For this review, take the finished solid that the model builds, in its own axes (mm). Face numbers are marked on the shaded views. A direction names the side the tool comes from. Coordinates: 2 decimals unless noted, no trailing zeros. Order: outer loops, then holes, each group sorted by start corner. A loop starts at its lowest first (then second) coordinate and runs counter-clockwise, first axis right, second up. Notation, with made-up numbers: (24, -14.5) -> (83, -14.5) arc R38 ccw to (83, 24.5) -> close; hole circle Ø2 at (87.5, -25.75). An arc over 180 degrees is marked (long way). Answer as a JSON object with one key per item and string values. Group by question number.
1) Wall thickness on L1, parallel to Y at x = -27.5, z = -1; L2, parallel to Y at x = -47.5, z = -0.75; L3, parallel to Z at x = -64, y = -17.5: over which ranges is each line inside the solid? List them lowest first.
2) Add section A-A, the plane x = -45. Write out the cut boundary in (y, z), then the cut area to 3 significant figures.
3) Add section B-B, the plane x = 8.5. Write out the cut boundary in (y, z).
4) Machinability: for the marked faces 1 and 2, which of the approach directions +Z, -Z, +X, -X, +Y, -Y give a long, thin tool a straight path to every point of the face, cutting with its end or side? Answer none if there is none.
5) Draft analysis for pull direction Y (two halves, no side actions). For the marked faces 3, 4 and 5, state which applies: +Y half, -Y half, draft (parallel to the pull), parting line (faces both ways), or undercut.
6) Add section C-C, the plane y = -19. Write out the cut boundary in (x, z).
7) For pin 1 (10.5 mm diameter, centred on x = -19.5, y = 22.5, fed in from +Z); pin 2 (1.6 mm diameter, centred on x = -50.5, z = -12.5, fed in from -Y); pin 3 (18.5 mm diameter, centred on x = 9, y = 35.5, fed in from -Z), all flat-tipped, find the tip position at first contact; note any pin that passes through.
8) Add section D-D, the plane x = -12. Write out the cut boundary in (y, z), then the cut area to 3 significant figures.
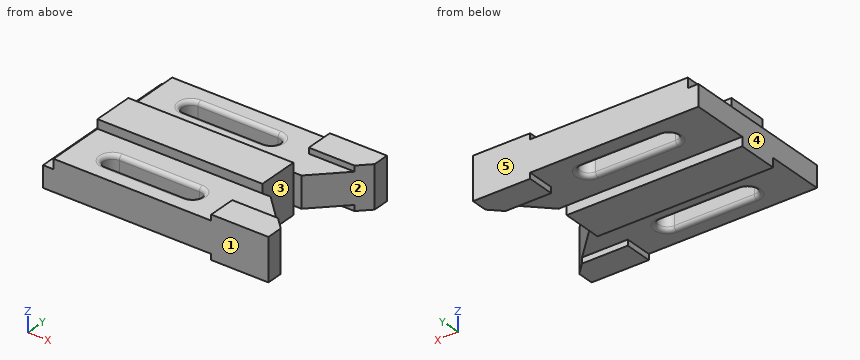
from build123d import *

# Parameters (mm, degrees)
EXTRUDE_1_DEPTH      = 9.5
EXTRUDE_2_DEPTH      = 3.5
EXTRUDE_2_DEPTH_BACK = 22.5
EXTRUDE_3_DEPTH      = 5.5
EXTRUDE_3_DEPTH_BACK = 24.5
SKETCH_8_W           = 107.5
SKETCH_8_H           = 25
SKETCH_9_W           = 6.5
SKETCH_9_H           = 96
CUT_EXTRUDE_1_DEPTH  = 11.5
CUT_EXTRUDE_2_DEPTH  = 52.5
FILLET_1_R           = 2.5


with BuildPart() as part:
    # 草图1 → 凸台-拉伸1 (new, symmetric)
    with BuildSketch(Plane.XY):
        Polygon((-107.5, 48), (30.5, 48), (30.5, 38), (5, 12.5), (0, 12.5), (0, -12.5), (5, -12.5), (30.5, -38), (30.5, -48), (-107.5, -48), align=None)
    extrude(amount=EXTRUDE_1_DEPTH, both=True)

    # 草图2 → 凸台-拉伸2 (add, two sides: drawn at the far end of the back side and taken through both)
    with BuildSketch(Plane.XY.offset(9.5).offset(-EXTRUDE_2_DEPTH_BACK)):
        Polygon((-4.5, 31), (23.5, 31), (30.5, 38), (30.5, 48), (-4.5, 48), align=None)
        Polygon((30.5, -38), (23.5, -31), (-4.5, -31), (-4.5, -48), (30.5, -48), align=None)
    extrude(amount=EXTRUDE_2_DEPTH + EXTRUDE_2_DEPTH_BACK)

    # 草图8 → 凸台-拉伸3 (add, two sides: drawn at the far end of the back side and taken through both)
    with BuildSketch(Plane(origin=(0, 0, -9.5), x_dir=(-1, 0, 0), z_dir=(0, 0, -1)).offset(-EXTRUDE_3_DEPTH_BACK)):
        with Locations((53.75, 0)):
            Rectangle(SKETCH_8_W, SKETCH_8_H)
    extrude(amount=EXTRUDE_3_DEPTH + EXTRUDE_3_DEPTH_BACK)

    # 草图9 → 切除-拉伸1 (cut)
    with BuildSketch(Plane.XY.offset(15)):
        with Locations((-104.25, 0)):
            Rectangle(SKETCH_9_W, SKETCH_9_H)
    extrude(amount=-CUT_EXTRUDE_1_DEPTH, mode=Mode.SUBTRACT)

    # 草图11 → 切除-拉伸2 (cut)
    with BuildSketch(Plane(origin=(0, 0, -9.5), x_dir=(-1, 0, 0), z_dir=(0, 0, -1))):
        with BuildLine():
            Line((28, 37.09009956), (77, 37.09009956))
            ThreePointArc((77, 37.09009956), (82.5, 31.59009956), (77, 26.09009956))
            Line((77, 26.09009956), (28, 26.09009956))
            ThreePointArc((28, 26.09009956), (22.5, 31.59009956), (28, 37.09009956))
        make_face()
        with BuildLine():
            Line((28, -26.570922994), (77, -26.570922994))
            ThreePointArc((77, -26.570922994), (82.5, -32.070922994), (77, -37.570922994))
            Line((77, -37.570922994), (28, -37.570922994))
            ThreePointArc((28, -37.570922994), (22.5, -32.070922994), (28, -26.570922994))
        make_face()
    extrude(amount=-CUT_EXTRUDE_2_DEPTH, mode=Mode.SUBTRACT)

    # 圆角1
    fillet_1_edges = [part.edges().sort_by_distance(p)[0] for p in [
        (-22.5, 31.59009956, 9.5),
        (-52.5, 37.09009956, 9.5),
        (-82.5, 31.59009956, 9.5),
        (-52.5, 26.09009956, 9.5),
        (-22.5, 31.59009956, -9.5),
        (-52.5, 26.09009956, -9.5),
        (-82.5, 31.59009956, -9.5),
        (-52.5, 37.09009956, -9.5),
        (-22.5, -32.070922994, 9.5),
        (-52.5, -26.570922994, 9.5),
        (-82.5, -32.070922994, 9.5),
        (-52.5, -37.570922994, 9.5),
        (-22.5, -32.070922994, -9.5),
        (-52.5, -37.570922994, -9.5),
        (-82.5, -32.070922994, -9.5),
        (-52.5, -26.570922994, -9.5),
    ]]
    fillet(fillet_1_edges, radius=FILLET_1_R)


solid = part.part
Output values:
{
 "1": {"L1": "y = -48 to -37.55, -26.59 to 26.11, 37.07 to 48", "L2": "y = -48 to -37.57, -26.57 to 26.09, 37.09 to 48", "L3": "z = -9.5 to 9.5"},
 "2": {"outline": "(-48, -9.5) -> (-40.07, -9.5) arc R2.5 ccw to (-37.57, -7) -> (-37.57, 7) arc R2.5 ccw to (-40.07, 9.5) -> (-48, 9.5) -> close; (-26.57, -7) arc R2.5 ccw to (-24.07, -9.5) -> (-12.5, -9.5) -> (-12.5, -15) -> (12.5, -15) -> (12.5, -9.5) -> (23.59, -9.5) arc R2.5 ccw to (26.09, -7) -> (26.09, 7) arc R2.5 ccw to (23.59, 9.5) -> (12.5, 9.5) -> (12.5, 15) -> (-12.5, 15) -> (-12.5, 9.5) -> (-24.07, 9.5) arc R2.5 ccw to (-26.57, 7) -> close; (37.09, -7) arc R2.5 ccw to (39.59, -9.5) -> (48, -9.5) -> (48, 9.5) -> (39.59, 9.5) arc R2.5 ccw to (37.09, 7) -> close", "area": "1,670 mm²"},
 "3": {"outline": "(-48, -13) -> (-31, -13) -> (-31, -9.5) -> (-16, -9.5) -> (-16, 9.5) -> (-31, 9.5) -> (-31, 13) -> (-48, 13) -> close; (16, -9.5) -> (31, -9.5) -> (31, -13) -> (48, -13) -> (48, 13) -> (31, 13) -> (31, 9.5) -> (16, 9.5) -> close"},
 "4": {"face 1": "+Z, -Z, +X, -X, -Y", "face 2": "+Z, -Z, +X"},
 "5": {"face 3": "undercut", "face 4": "draft", "face 5": "+Y half"},
 "6": {"outline": "(-107.5, -9.5) -> (11.5, -9.5) -> (11.5, 9.5) -> (-101, 9.5) -> (-101, 3.5) -> (-107.5, 3.5) -> close"},
 "7": {"pin 1": "stops at z = 9.5", "pin 2": "stops at y = -12.5", "pin 3": "stops at z = -13"},
 "8": {"outline": "(-48, -9.5) -> (-12.5, -9.5) -> (-12.5, -15) -> (12.5, -15) -> (12.5, -9.5) -> (48, -9.5) -> (48, 9.5) -> (12.5, 9.5) -> (12.5, 15) -> (-12.5, 15) -> (-12.5, 9.5) -> (-48, 9.5) -> close", "area": "2,100 mm²"}
}
